from build123d import *

# Parameters (mm, degrees)
SKETCH1_W             = 41.656
SKETCH1_H             = 16.51
BOSS_EXTRUDE1_DEPTH   = 6.35
SKETCH2_W             = 2.54
SKETCH2_H             = 16.51
BOSS_EXTRUDE2_DEPTH   = 2.54
SKETCH3_W             = 2.54
SKETCH3_H             = 16.51
BOSS_EXTRUDE3_DEPTH   = 5.08
F_3_0MM_DOWEL_HOLE1_D = 3
FILLET1_R             = 1.27
CHAMFER1_SIZE         = 0.254
FILLET2_R             = 3.81


# Some blends are built 0.0001 mm under size
with BuildPart() as part:
    # Sketch1 → Boss-Extrude1 (new body)
    with BuildSketch(Plane(origin=(0, 0, 0), x_dir=(1, 0, 0), z_dir=(0, 1, 0))):
        with Locations((20.828, 8.255)):
            Rectangle(SKETCH1_W, SKETCH1_H)
    extrude(amount=BOSS_EXTRUDE1_DEPTH)

    # Sketch2 → Boss-Extrude2 (add)
    with BuildSketch(Plane.XZ):
        with Locations((37.846, -8.255)):
            Rectangle(SKETCH2_W, SKETCH2_H)
    extrude(amount=BOSS_EXTRUDE2_DEPTH)

    # Sketch3 → Boss-Extrude3 (add)
    with BuildSketch(Plane.XZ):
        with Locations((19.05, -8.255)):
            Rectangle(SKETCH3_W, SKETCH3_H)
    extrude(amount=BOSS_EXTRUDE3_DEPTH)

    # Ø3.0mm Dowel Hole1 (through all)
    with Locations(Plane(origin=(0, 6.35, 0), x_dir=(1, 0, 0), z_dir=(0, 1, 0))):
        with Locations((5.08, 8.255), (12.7, 8.255)):
            Hole(F_3_0MM_DOWEL_HOLE1_D / 2)

    # Fillet1
    fillet1_edges = [part.edges().sort_by_distance(p)[0] for p in [
        (41.656, 6.35, -8.255),
        (20.828, 6.35, -16.51),
        (28.448, 0, -16.51),
        (40.386, 0, 0),
        (39.116, 0, -8.255),
        (39.116, -1.27, -16.51),
        (39.116, -1.27, 0),
        (36.576, 0, -8.255),
        (36.576, -1.27, 0),
        (36.576, -1.27, -16.51),
        (39.116, -2.54, -8.255),
        (36.576, -2.54, -8.255),
        (28.448, 0, 0),
        (8.89, 0, -16.51),
        (20.32, 0, -8.255),
        (20.32, -2.54, -16.51),
        (20.32, -2.54, 0),
        (17.78, 0, -8.255),
        (17.78, -2.54, 0),
        (17.78, -2.54, -16.51),
        (20.32, -5.08, -8.255),
        (19.05, -5.08, 0),
        (17.78, -5.08, -8.255),
        (19.05, -5.08, -16.51),
        (0, 6.35, -8.255),
        (40.386, 0, -16.51),
        (41.656, 0, -8.255),
        (8.89, 0, 0),
        (0, 0, -8.255),
        (20.828, 6.35, 0),
        (41.656, 3.175, -16.51),
        (41.656, 3.175, 0),
    ]]
    fillet(fillet1_edges, radius=FILLET1_R - 0.0001)  # a hair under: the kernel refuses the full size

    # Chamfer1
    chamfer1_edges = [part.edges().sort_by_distance(p)[0] for p in [
        (14.2, 0, -8.255),
        (14.2, 6.35, -8.255),
        (6.58, 0, -8.255),
        (6.58, 6.35, -8.255),
    ]]
    chamfer(chamfer1_edges, length=CHAMFER1_SIZE)

    # Fillet2
    # the kernel refuses this fillet: 3.81 mm, written as the material it takes off along each edge
    with BuildSketch(Plane(origin=(3.81, 0, -3.81), x_dir=(0, 0, 1), z_dir=(1, 0, 0))) as fillet2_piece_1:
        with BuildLine():
            CenterArc((2.5401, -1.2699), 1.2699, 0, 90)
            Line((3.81, -1.2699), (3.81, 0))
            Line((3.81, 0), (2.5401, 0))
        make_face()
    revolve(axis=Axis((3.81, 0, -3.81), (0, -1, 0)), revolution_arc=90, mode=Mode.SUBTRACT)
    with BuildSketch(Plane(origin=(3.81, 0, -12.7), x_dir=(-1, 0, 0), z_dir=(0, 0, 1))) as fillet2_piece_2:
        with BuildLine():
            CenterArc((2.5401, -1.2699), 1.2699, 0, 90)
            Line((3.81, -1.2699), (3.81, 0))
            Line((3.81, 0), (2.5401, 0))
        make_face()
    revolve(axis=Axis((3.81, 0, -12.7), (0, -1, 0)), revolution_arc=90, mode=Mode.SUBTRACT)
    with BuildSketch(Plane(origin=(3.81, 6.35, -3.81), x_dir=(-1, 0, 0), z_dir=(0, 0, -1))) as fillet2_piece_3:
        with BuildLine():
            CenterArc((2.5401, -1.2699), 1.2699, 0, 90)
            Line((3.81, -1.2699), (3.81, 0))
            Line((3.81, 0), (2.5401, 0))
        make_face()
    revolve(axis=Axis((3.81, 6.35, -3.81), (0, 1, 0)), revolution_arc=90, mode=Mode.SUBTRACT)
    with BuildSketch(Plane(origin=(3.81, 6.35, -12.7), x_dir=(0, 0, -1), z_dir=(1, 0, 0))) as fillet2_piece_4:
        with BuildLine():
            CenterArc((2.5401, -1.2699), 1.2699, 0, 90)
            Line((3.81, -1.2699), (3.81, 0))
            Line((3.81, 0), (2.5401, 0))
        make_face()
    revolve(axis=Axis((3.81, 6.35, -12.7), (0, 1, 0)), revolution_arc=90, mode=Mode.SUBTRACT)
    with BuildSketch(Plane(origin=(0, 0, -16.51), x_dir=(1, 0, 0), z_dir=(0, 1, 0)), Plane(origin=(0, 0, 0), x_dir=(0, 0, -1), z_dir=(0, 1, 0))) as fillet2_piece_5:
        with BuildLine():
            CenterArc((FILLET2_R, -FILLET2_R), FILLET2_R, 90, 90)
            Line((0, -FILLET2_R), (0, 0))
            Line((0, 0), (FILLET2_R, 0))
        make_face()
    extrude(amount=6.35, mode=Mode.SUBTRACT)


solid = part.part
Read the model definition and answer for the solid it produces. Units are mm, in the model's axes. A direction names the side the tool comes from. Round coordinates to 2 decimals unless told otherwise and drop trailing zeros. Write each loop counter-clockwise with the first axis right and the second up, starting at its lowest first coordinate (ties: lowest second). Pieces come first, ordered by that corner, then holes.
Q1. A tool of negligible diameter and unlimited length cuts with its end or side. For faces 1 (the face through (17.78, -3, -8)), 2 (the face through (10.249, 0.382, -16.148)), 3 (the face through (20.32, -3, -8)), 4 (the face through (38.56, -1.77, -0.22)), from which of +Z, -Z, +X, -X, +Y, -Y can it reach the whole face along a straight path? Write none if from no direction.
Values:
face 1: +Z, -Z, -X, -Y
face 2: -Z, -X, -Y
face 3: +Z, -Z, -Y
face 4: +Z, +X, -Y
Q2. Find section A-A on x = 5.08. Determine the outline of the cut face in (y, z) (3 decimals).
Values:
outline: (0, -15.24) arc R1.27 ccw to (1.27, -16.51) - (5.08, -16.51) arc R1.27 ccw to (6.35, -15.24) - (6.35, -10.009) - (6.096, -9.755) - (0.254, -9.755) - (0, -10.009) - close; (0, -6.501) - (0.254, -6.755) - (6.096, -6.755) - (6.35, -6.501) - (6.35, -1.27) arc R1.27 ccw to (5.08, 0) - (1.27, 0) arc R1.27 ccw to (0, -1.27) - close
Q3. Find section C-C on y = 2.5. Determine the outline of the cut face in (x, z) (3 decimals).
Values:
outline: (0, -12.7) arc R3.81 ccw to (3.81, -16.51) - (40.386, -16.51) arc R1.27 ccw to (41.656, -15.24) - (41.656, -1.27) arc R1.27 ccw to (40.386, 0) - (3.81, 0) arc R3.81 ccw to (0, -3.81) - close; hole circle Ø3 at (5.08, -8.255); hole circle Ø3 at (12.7, -8.255)
Q4. Straight lines are drawn through the part: line 1 (Z direction, x = 5.08, y = 3.45) (3 decimals); line 2 (Y direction, x = 22, z = -15); line 3 (X direction, y = 3, z = -8.5). For each, find the intervals that lie inside material, in ascending order.
Values:
line 1: z = -16.51 to -9.755, -6.755 to 0
line 2: y = 0 to 6.35
line 3: x = 0 to 3.6, 6.56 to 11.22, 14.18 to 41.66
Q5. The mould has two halves that part along Z. Classify faces 5 (the face through (11.314, 3.134, -7.68)), 6 (the face through (1.146, 3.148, -15.424)), 7 (the face through (38.75, -2.16, -8.14)): released by +Z, released by -Z, zero draft, split by the parting line, or undercut.
Values:
face 5: undercut
face 6: released by -Z
face 7: zero draft
Q6. Flat-ended cylindrical pins translate along their axes: P1, Ø4, axis at x = 36, y = -3.5, coming from the -Z side; P2, Ø1, axis at x = 27.5, y = 0, coming from the -Z side; P3, Ø7, axis at x = 26, z = -10.5, coming from the -Y side. Find the tip coordinate at first contact, or state that the pin passes through.
Values:
P1: stops at z = -16.51
P2: stops at z = -16.25
P3: stops at y = 0
Q7. Find section D-D on x = 33. Determine the outline of the cut face in (y, z), and give its area (3 significant figures).
Values:
outline: (0, -15.24) arc R1.27 ccw to (1.27, -16.51) - (5.08, -16.51) arc R1.27 ccw to (6.35, -15.24) - (6.35, -1.27) arc R1.27 ccw to (5.08, 0) - (1.27, 0) arc R1.27 ccw to (0, -1.27) - close
area: 103 mm2
